Autodesk Inventor part; units mm, degrees
ref_plane "YZ Plane" through (0, 0, 0) normal (1, 0, 0) x (0, 1, 0)
ref_plane "XZ Plane" through (0, 0, 0) normal (0, 1, 0) x (-1, 0, 0)
ref_plane "XY Plane" through (0, 0, 0) normal (0, 0, 1) x (1, 0, 0)
sketch "Sketch1" plane through (0, 0, 0) normal (0, 1, 0) x (-1, 0, 0)
  circle A0 centre (0, 0) radius 4.5
  dimension "d0" = 9
extrude "Extrusion1" add sketch "Sketch1" along normal blind 2
sketch "Sketch2" plane through (0, 2, 0) normal (0, 1, 0) x (1, 0, 0)
  circle A0 centre (0, 0) radius 2.75
  dimension "d3" = 5.5
extrude "Extrusion2" add sketch "Sketch2" along normal blind 60
chamfer "Chamfer1" distance 2.7 angle 45 1 edges at (-2.75, 62, 0)
properties part number "Fan_Pin"
Here's how the part is built. I have some questions about the finished solid (model axes, mm). A direction names the side the tool comes from. Give positions to 0.01 mm unless a question says otherwise; leave off trailing zeros. Order: outer loops, then holes, each group sorted by start corner. A loop starts at its lowest first (then second) coordinate and runs counter-clockwise, first axis right, second up. Notation, with made-up numbers: (80.5, -2.5) - (105.5, -2.5) arc R24 cw to (105.5, 18.5) - close; hole circle Ø8 at (-3, 26). An arc over 180 degrees is marked (long way). Answer as a JSON object with one key per item and string values. Group by question number.
Item 1: Which directions (+Z, -Z, +X, -X, +Y, -Y) give clear straight access to the entire face, cutting with the end or side of a thin tool? Please do faces 1 (the cylindrical face through (0.59, 0.99, -4.46)), 2 (the flat face through (0, 2, -3)).
Item 2: If we section it at A-A on y = 12: Please give me the cut outline in (x, z).
Item 3: If we section it at C-C on x = 3.5: Please give me the cut outline in (y, z).
Item 4: For P1, Ø1.5, axis at x = -2, y = 10, coming from the +Z side; P2, Ø5, axis at x = -3.5, y = 42.5, coming from the +Z side; P3, Ø1, axis at x = 1, y = 11.5, coming from the -Z side; P4, Ø4, axis at x = -0.5, z = 1.5, coming from the +Y side, each with a flat end and sliding along its axis, tell me the tip position at first contact or that it passes through.
Item 5: Please list where these lines run through material, in increasing order: probe 1 along Y at (x, z) = (2, 2); probe 2 along X at (y, z) = (4, 0); probe 3 along Z at (x, y) = (1.5, 13.5).
Item 6: If we section it at B-B on z = -3.5: Please give me the cut outline in (x, y), and give its area (3 significant figures).
Result set:
{
 "1": {"face 1": "+Y, -Y", "face 2": "+Y"},
 "2": {"outline": "circle Ø5.5 at (0, 0)"},
 "3": {"outline": "(0, -2.83) - (2, -2.83) - (2, 2.83) - (0, 2.83) - close"},
 "4": {"P1": "z = 2.45", "P2": "z = 2.56", "P3": "z = -2.7", "P4": "y = 62"},
 "5": {"probe 1": "0 to 2", "probe 2": "-2.75 to 2.75", "probe 3": "-2.3 to 2.3"},
 "6": {"outline": "(-2.83, 0) - (2.83, 0) - (2.83, 2) - (-2.83, 2) - close", "area": "11.3 mm²"}
}
